Read the model definition and answer for the solid it produces. Units are mm, in the model's axes. Face numbers are marked on the shaded views. A direction names the side the tool comes from. Coordinates: 2 decimals unless noted, no trailing zeros. Write each loop counter-clockwise with the first axis right and the second up, starting at its lowest first coordinate (ties: lowest second). Pieces come first, ordered by that corner, then holes. Notation, with made-up numbers: (-3.5, 64) - (53.5, 64) arc R28 cw to (53.5, 85) - close; hole circle Ø4 at (28.5, 27). An arc over 180 degrees is marked (long way). Use a Markdown table: item, result.
Autodesk Inventor part; units mm, degrees
ref_plane "YZ Plane" through (0, 0, 0) normal (1, 0, 0) x (0, 1, 0)
ref_plane "XZ Plane" through (0, 0, 0) normal (0, 1, 0) x (-1, 0, 0)
ref_plane "XY Plane" through (0, 0, 0) normal (0, 0, 1) x (1, 0, 0)
sketch "Sketch1" plane through (0, 0, 0) normal (0, 0, 1) x (1, 0, 0)
  line L0 (-6.35, 31.75) -> (-6.35, 0)
  line L1 (-6.35, 0) -> (6.35, 0)
  line L2 (6.35, 0) -> (6.35, 31.75)
  arc A0 (6.35, 31.75) -> (-6.35, 31.75) centre (0, 23.8189) ccw
  point P0 (0, 0)
  dimension "d1" = 31.75
  dimension "d2" = 12.7
  dimension "d3" = 10.16
extrude "Extrusion1" add sketch "Sketch1" along normal mid plane 38.1
sketch "Sketch2" plane through (0, 0, 0) normal (0, 0, 1) x (1, 0, 0)
  line L0 (-6.35, 0) -> (6.35, 0)
  line L1 (6.35, 0) -> (6.35, 12.7)
  line L2 (6.35, 12.7) -> (-6.35, 12.7)
  line L3 (-6.35, 12.7) -> (-6.35, 0)
  line L4 (0, -2.54) -> (0, 15.24)
  point P0 (0, 0)
  dimension "d6" = 12.7
  dimension "d7" = 6.35
  dimension "d10" = 12.7
extrude "Extrusion2" cut sketch "Sketch2" along normal mid plane 25.4
fillet "Fillet1" radius 3.175 2 edges at (-6.35, 12.7, 0) (6.35, 12.7, 0)
equation "\"d7\" = 0.5 * d6"
properties part number "Odyssey Bushing"
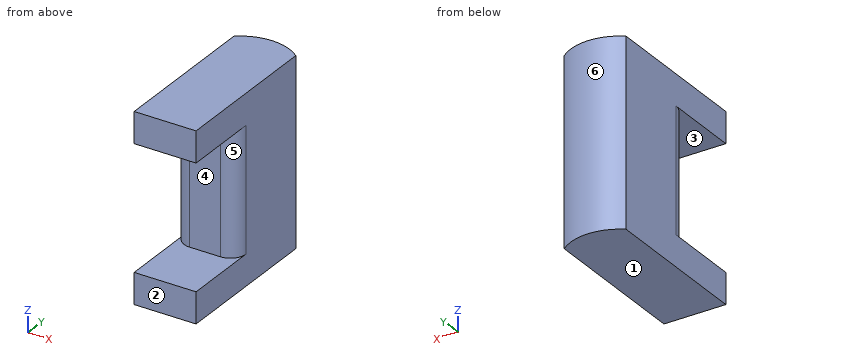
(1) For the marked faces 4, 5 and 6, determine the directions among +Z, -Z, +X, -X, +Y, -Y from which every point of the face is accessible in a straight line to the end or side of a thin tool.
Report:
| item | result |
|---|---|
| face 4 | +X, -X, -Y |
| face 5 | +X, -Y |
| face 6 | +Z, -Z, +Y |
(2) A cutting plane is placed at D-D, the plane y = 14. Write down the section's boundary in (x, z), and give its area (3 significant figures).
Report:
| item | result |
|---|---|
| outline | (-6.35, -19.05) - (6.35, -19.05) - (6.35, -12.7) - (5.74, -12.7) - (5.74, 12.7) - (6.35, 12.7) - (6.35, 19.05) - (-6.35, 19.05) - (-6.35, 12.7) - (-5.74, 12.7) - (-5.74, -12.7) - (-6.35, -12.7) - close |
| area | 453 mm² |
(3) Each of these flat-tipped pins is pushed along its axis until it touches: P1, Ø3, axis at x = -0.5, z = -1, coming from the -Y side; P2, Ø1.5, axis at y = 13, z = 3.5, coming from the -X side. Where does it stop, or does it pass through?
Report:
| item | result |
|---|---|
| P1 | stops at y = 12.7 |
| P2 | stops at x = -5.53 |
(4) The mould has two halves that part along Z. Classify the marked faces 1, 2 and 3: pulls with the +Z half, pulls with the -Z half, needs draft (parallel to the pull), parting line crosses it, or undercut.
Report:
| item | result |
|---|---|
| face 1 | pulls with the -Z half |
| face 2 | needs draft |
| face 3 | undercut |
(5) A cutting plane is placed at B-B, the plane z = 5. Write down the section's boundary in (x, y) (3 decimals), and give its area (3 significant figures).
Report:
| item | result |
|---|---|
| outline | (-6.35, 15.875) arc R3.175 ccw to (-3.175, 12.7) - (3.175, 12.7) arc R3.175 ccw to (6.35, 15.875) - (6.35, 31.75) arc R10.16 ccw to (-6.35, 31.75) - close |
| area | 257 mm² |
(6) A cutting plane is placed at A-A, the plane y = 9.5. Write down the section's boundary in (x, z).
Report:
| item | result |
|---|---|
| outline | (-6.35, -19.05) - (6.35, -19.05) - (6.35, -12.7) - (-6.35, -12.7) - close; (-6.35, 12.7) - (6.35, 12.7) - (6.35, 19.05) - (-6.35, 19.05) - close |
(7) A cutting plane is placed at C-C, the plane x = -0.75. Write down the section's boundary in (y, z), and give its area (3 significant figures).
Report:
| item | result |
|---|---|
| outline | (0, -19.05) - (33.95, -19.05) - (33.95, 19.05) - (0, 19.05) - (0, 12.7) - (12.7, 12.7) - (12.7, -12.7) - (0, -12.7) - close |
| area | 971 mm² |
(8) Straight lines are drawn through the part: L1, parallel to Z at x = 5, y = 4.5; L2, parallel to X at y = 14, z = -11.5; L3, parallel to Y at x = 4.5, z = -17. For each, find the intervals that lie inside material, in ascending order.
Report:
| item | result |
|---|---|
| L1 | z = -19.05 to -12.7, 12.7 to 19.05 |
| L2 | x = -5.74 to 5.74 |
| L3 | y = 0 to 32.93 |
